Design review of the part built by this model. Coordinates are the model's own, in mm. A direction names the side the tool comes from. Give positions to 0.01 mm unless a question says otherwise; leave off trailing zeros. Order: outer loops, then holes, each group sorted by start corner. A loop starts at its lowest first (then second) coordinate and runs counter-clockwise, first axis right, second up. Notation, with made-up numbers: (57, -21.5) -> (87, -21.5) arc R6 cw to (87, -10.5) -> close; hole circle Ø5 at (28, 59.5). An arc over 180 degrees is marked (long way). One line per item, written item: value.
from build123d import *

# Parameters (mm, degrees)
SKETCH1_W           = 3.38
SKETCH1_H           = 4
BOSS_EXTRUDE1_DEPTH = 1.82
SKETCH2_W           = 1
SKETCH2_H           = 1
BOSS_EXTRUDE2_DEPTH = 6.82


with BuildPart() as part:
    # Sketch1 → Boss-Extrude1 (new body)
    with BuildSketch(Plane(origin=(0, 0, 0), x_dir=(1, 0, 0), z_dir=(0, 1, 0))):
        with Locations((1.69, 2)):
            Rectangle(SKETCH1_W, SKETCH1_H)
    extrude(amount=BOSS_EXTRUDE1_DEPTH)

    # Sketch2 → Boss-Extrude2 (add)
    with BuildSketch(Plane.XY):
        with Locations((0.9, 0.91)):
            Rectangle(SKETCH2_W, SKETCH2_H)
        with Locations((2.48, 0.91)):
            Rectangle(SKETCH2_W, SKETCH2_H)
    extrude(amount=BOSS_EXTRUDE2_DEPTH)


solid = part.part
Item 1: Machinability: for faces 1 (the flat face through (1, 1, 6.82)), 2 (the flat face through (1, 0.41, 3)), 3 (the flat face through (2.98, 1, 3)), 4 (the flat face through (1, 1.41, 3)), which of the approach directions +Z, -Z, +X, -X, +Y, -Y give a long, thin tool a straight path to every point of the face, cutting with its end or side? Answer none if there is none.
Returned:
face 1: +Z, +X, -X, +Y, -Y
face 2: +Z, +X, -X, -Y
face 3: +Z, +X, +Y, -Y
face 4: +Z, +X, -X, +Y
Item 2: To check wall thickness, follow line 1 along X through (y, z) = (1.3, 3); line 2 along Z through (x, y) = (2.75, 1.55); line 3 along Y through (x, z) = (0.45, 3.25). State the ranges of each line that lie inside material, in increasing order. Write a range as from..to.
Returned:
line 1: 0.4..1.4, 1.98..2.98
line 2: -4..0
line 3: 0.41..1.41
Item 3: Add section D-D on y = 0.2. Give the boundary of the cut face in (x, z).
Returned:
outline: (0, -4) -> (3.38, -4) -> (3.38, 0) -> (0, 0) -> close
Item 4: Add section C-C on x = 2.65. Give the boundary of the cut face in (y, z), plus the area to 3 significant figures.
Returned:
outline: (0, -4) -> (1.82, -4) -> (1.82, 0) -> (1.41, 0) -> (1.41, 6.82) -> (0.41, 6.82) -> (0.41, 0) -> (0, 0) -> close
area: 14.1 mm²
Item 5: Clearance check with flat-ended pins moving along their axes: P1, Ø2, axis at x = 3, z = 2.5, coming from the +Y side; P2, Ø0.8, axis at y = 1, z = 4.5, coming from the -X side; P3, Ø0.5, axis at x = 2.5, z = 3.5, coming from the -Y side. State where each tip first meets the part, or that it passes through.
Returned:
P1: y = 1.41
P2: x = 0.4
P3: y = 0.41
Item 6: Draft analysis for pull direction X (two halves, no side actions). For faces 5 (the flat face through (2, 0, -2)), 6 (the flat face through (1.4, 1, 3)), 7 (the flat face through (1.98, 1, 3)), 8 (the flat face through (0.4, 1, 3)), state which applies: pulls with the +X half, pulls with the -X half, needs draft (parallel to the pull), parting line crosses it, or undercut.
Returned:
face 5: needs draft
face 6: undercut
face 7: undercut
face 8: pulls with the -X half
Item 7: Add section B-B on y = 1.3. Give the boundary of the cut face in (x, z).
Returned:
outline: (0, -4) -> (3.38, -4) -> (3.38, 0) -> (2.98, 0) -> (2.98, 6.82) -> (1.98, 6.82) -> (1.98, 0) -> (1.4, 0) -> (1.4, 6.82) -> (0.4, 6.82) -> (0.4, 0) -> (0, 0) -> close
Item 8: Add section A-A on z = 0.75. Give the boundary of the cut face in (x, y), plus the area to 3 significant figures.
Returned:
outline: (0.4, 0.41) -> (1.4, 0.41) -> (1.4, 1.41) -> (0.4, 1.41) -> close; (1.98, 0.41) -> (2.98, 0.41) -> (2.98, 1.41) -> (1.98, 1.41) -> close
area: 2.00 mm²
